Geometry: final body of the model. Coordinates: model frame, mm. A direction names the side the tool comes from. Round coordinates to 2 decimals unless told otherwise and drop trailing zeros. Write each loop counter-clockwise with the first axis right and the second up, starting at its lowest first coordinate (ties: lowest second). Pieces come first, ordered by that corner, then holes. Notation, with made-up numbers: (48.25, 25.5) - (104.25, 25.5) arc R20 ccw to (104.25, 43.5) - close; hole circle Ø11 at (40, 38). An arc over 180 degrees is marked (long way). Use a Markdown table: item, result. Add a question column.
```python
from build123d import *

# Parameters (mm, degrees)
CHAMFER_2_SIZE           = 1.25
CHAMFER_2_SIZE2          = 0.334936491
CHAMFER_3_SIZE           = 1.25
CHAMFER_3_SIZE2          = 0.334936491
SKETCH_4_R               = 2
CUT_EXTRUDE_2_DEPTH      = 1
CUT_EXTRUDE_2_DEPTH_BACK = 7


with BuildPart() as part:
    # Эскиз2 → Повернуть2 (revolve)
    with BuildSketch(Plane.XY):
        Polygon((0, 0), (6.75, 0), (6.75, 3), (3, 3), (3, 6), (0, 6), align=None)
    revolve(axis=Axis((0, 6, 0), (0, -1, 0)))

    # Фаска2
    chamfer_2_edges = [part.edges().sort_by_distance(p)[0] for p in [
        (-6.75, 3, 0),
    ]]
    chamfer_2_side = [part.faces().sort_by_distance(p)[0] for p in [
        (-6.559081169, 3, 0),
    ]]
    chamfer(chamfer_2_edges, length=CHAMFER_2_SIZE, length2=CHAMFER_2_SIZE2, reference=chamfer_2_side[0])

    # Фаска3
    chamfer_3_edges = [part.edges().sort_by_distance(p)[0] for p in [
        (-6.75, 0, 0),
    ]]
    chamfer_3_side = [part.faces().sort_by_distance(p)[0] for p in [
        (0, 0, 0),
    ]]
    chamfer(chamfer_3_edges, length=CHAMFER_3_SIZE, length2=CHAMFER_3_SIZE2, reference=chamfer_3_side[0])

    # Эскиз4 → Вырез-Вытянуть2 (cut, two sides)
    with BuildSketch(Plane(origin=(0, 6, 0), x_dir=(1, 0, 0), z_dir=(0, 1, 0))) as cut_extrude_2_sk:
        Circle(SKETCH_4_R)
    extrude(amount=CUT_EXTRUDE_2_DEPTH, mode=Mode.SUBTRACT)
    extrude(cut_extrude_2_sk.sketch, amount=-CUT_EXTRUDE_2_DEPTH_BACK, mode=Mode.SUBTRACT)


solid = part.part
```
1) Section B-B, the plane x = 0. Return the cut outline in (y, z).
2) Draft query along Z for faces 1 (the cylindrical face through (-1.46, 1.52, -6.59)), 2 (the cylindrical face through (0, 3, 2)), 3 (the flat face through (1, 6, -2)). Return one class per face: released by +Z, released by -Z, zero draft, split by the parting line, or undercut.
3) Set-up query: faces 4 (the flat face through (2.4, 3, -2.4)), 5 (the flat face through (0.1, 0, -2.4)). Return all of +Z, -Z, +X, -X, +Y, -Y with unobstructed straight access to the full face (end or side cutting, diameter ignored); none if empty.
4) Section C-C, the plane y = 0.75. Return the cut outline in (x, z), then the cut area to 3 significant figures.
5) Pin query (flat end, axial travel): P1, Ø1, axis at x = -1.5, y = 5, coming from the -Z side; P2, Ø2, axis at x = -1, y = 5, coming from the -Z side; P3, Ø2, axis at y = 1.5, z = 2.5, coming from the +X side. Return the tip coordinate at first contact, or that it passes through.
6) Material intervals for L1, parallel to Z at x = 0, y = 2.4; L2, parallel to Z at x = 0, y = 3.45; L3, parallel to Y at x = -0.5, z = 3.25, sorted ascending. Write a range as from..to.
7) Section A-A, the plane z = 0. Return the cut outline in (x, y), then the cut area to 3 significant figures.
8) Section D-D, the plane y = 3.2. Return the cut outline in (x, z), then the cut area to 3 significant figures.
Output values:
| question | item | result |
|---|---|---|
| 1 | outline | (0, -5.5) - (0.33, -6.75) - (2.67, -6.75) - (3, -5.5) - (3, -3) - (6, -3) - (6, -2) - (0, -2) - close; (0, 2) - (6, 2) - (6, 3) - (3, 3) - (3, 5.5) - (2.67, 6.75) - (0.33, 6.75) - (0, 5.5) - close |
| 2 | face 1 | split by the parting line |
| 2 | face 2 | undercut |
| 2 | face 3 | zero draft |
| 3 | face 4 | +Y |
| 3 | face 5 | +Z, -Z, +X, -X, -Y |
| 4 | outline | circle Ø13.5 at (0, 0); hole circle Ø4 at (0, 0) |
| 4 | area | 131 mm^2 |
| 5 | P1 | stops at z = -2.83 |
| 5 | P2 | stops at z = -3 |
| 5 | P3 | stops at x = 6.58 |
| 6 | L1 | z = -6.75..-2, 2..6.75 |
| 6 | L2 | z = -3..-2, 2..3 |
| 6 | L3 | y = 0..3 |
| 7 | outline | (-6.75, 0.33) - (-5.5, 0) - (-2, 0) - (-2, 6) - (-3, 6) - (-3, 3) - (-5.5, 3) - (-6.75, 2.67) - close; (2, 0) - (5.5, 0) - (6.75, 0.33) - (6.75, 2.67) - (5.5, 3) - (3, 3) - (3, 6) - (2, 6) - close |
| 7 | area | 33.7 mm^2 |
| 8 | outline | circle Ø6 at (0, 0); hole circle Ø4 at (0, 0) |
| 8 | area | 15.7 mm^2 |
